from build123d import *

# Parameters (mm, degrees)
SKETCH_1_W      = 25
SKETCH_1_H      = 10
EXTRUDE_1_DEPTH = 3
FILLET_1_R      = 5


with BuildPart() as part:
    # 草图1 → 凸台-拉伸1 (new body)
    with BuildSketch(Plane(origin=(0, 0, 0), x_dir=(1, 0, 0), z_dir=(0, 1, 0))):
        with Locations((-7.5, 0)):
            Rectangle(SKETCH_1_W, SKETCH_1_H)
        with BuildLine():
            Line((0, -1.6), (-15, -1.6))
            ThreePointArc((-15, -1.6), (-16.6, 0), (-15, 1.6))
            Line((-15, 1.6), (0, 1.6))
            ThreePointArc((0, 1.6), (1.6, 0), (0, -1.6))
        make_face(mode=Mode.SUBTRACT)
    extrude(amount=EXTRUDE_1_DEPTH)

    # 圆角1
    fillet_1_edges = [part.edges().sort_by_distance(p)[0] for p in [
        (5, 1.5, 5),
        (5, 1.5, -5),
        (-20, 1.5, -5),
        (-20, 1.5, 5),
    ]]
    fillet(fillet_1_edges, radius=FILLET_1_R - 0.0001)  # a hair under: the kernel refuses the full size


solid = part.part
Geometry check sheet. Reference: the model listing, model coordinates, mm. A direction names the side the tool comes from. Coordinates: 2 decimals unless noted, no trailing zeros. Order: outer loops, then holes, each group sorted by start corner. A loop starts at its lowest first (then second) coordinate and runs counter-clockwise, first axis right, second up. Notation, with made-up numbers: (88, 10.5) - (119, 10.5) arc R19 cw to (119, 47.5) - close; hole circle Ø6 at (-2.5, -3). An arc over 180 degrees is marked (long way). Answer in a Markdown table with one row per item. Add a question column.
1) Cross-section at A-A, the plane x = -14.5. Record the cut outline in (y, z), then the cut area to 3 significant figures.
2) Cross-section at D-D, the plane z = 3.75. Record the cut outline in (x, y).
3) Material ranges on line 1 along Z through (x, y) = (-2, 2.5); line 2 along X through (y, z) = (2.35, 0); line 3 along X through (y, z) = (2.05, 0.5), recorded low to high. Write a range as [from, to].
4) Release check for a two-part mould opening along X. For faces 1 (the cylindrical face through (-19, 2, 3)), 2 (the flat face through (-7, 1, 1.6)), 3 (the cylindrical face through (3, 2, -4)) record: +X half, -X half, draft (parallel to the pull), parting line (faces both ways), or undercut.
5) Gauge pin test, flat end, axial feed: P1, Ø1.5, axis at y = 1, z = 3.5, coming from the -X side. Record the tip position at first contact, or that the pin passes through.
6) Set-up check for faces 4 (the cylindrical face through (-16.6, 1.5, 0)), 5 (the cylindrical face through (3, 2, 4)): record each of +Z, -Z, +X, -X, +Y, -Y from which the full face is reachable in a straight line by a thin tool's end or side.
7) Cross-section at C-C, the plane z = 1.25. Record the cut outline in (x, y), then the cut area to 3 significant figures.
Check result:
| question | item | result |
|---|---|---|
| 1 | outline | (0, -5) - (3, -5) - (3, -1.6) - (0, -1.6) - close; (0, 1.6) - (3, 1.6) - (3, 5) - (0, 5) - close |
| 1 | area | 20.4 mm² |
| 2 | outline | (-18.31, 0) - (3.31, 0) - (3.31, 3) - (-18.31, 3) - close |
| 3 | line 1 | z = [-5, -1.6], [1.6, 5] |
| 3 | line 2 | x = [-20, -16.6], [1.6, 5] |
| 3 | line 3 | x = [-19.97, -16.52], [1.52, 4.97] |
| 4 | face 1 | -X half |
| 4 | face 2 | undercut |
| 4 | face 3 | +X half |
| 5 | P1 | stops at x = -19.18 |
| 6 | face 4 | +Y, -Y |
| 6 | face 5 | +Z, +X, +Y, -Y |
| 7 | outline | (-19.84, 0) - (-16, 0) - (-16, 3) - (-19.84, 3) - close; (1, 0) - (4.84, 0) - (4.84, 3) - (1, 3) - close |
| 7 | area | 23.1 mm² |
